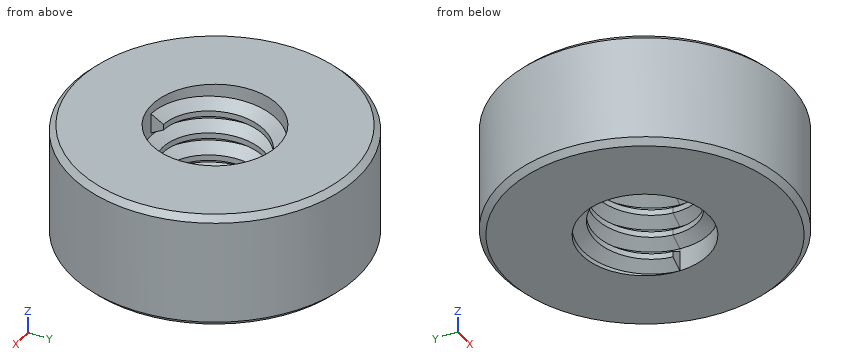
from build123d import *

# Parameters (mm, degrees)
SKETCH_1_R        = 2.5
EXTRUDE_1_DEPTH   = 2
CHAMFER_2_SIZE    = 0.1
HOLE_WIZARD_M21_D = 2.2
THREAD_1_PITCH    = 0.4
SCALE_1_SCALE     = 2


with BuildPart() as part:
    # Sketch 1 → Бобышка-Вытянуть1 (new body)
    with BuildSketch(Plane.XY):
        Circle(SKETCH_1_R)
    extrude(amount=EXTRUDE_1_DEPTH)

    # Фаска2
    chamfer_2_edges = [part.edges().sort_by_distance(p)[0] for p in [
        (-2.5, 0, 0),
        (-2.5, 0, 2),
    ]]
    chamfer(chamfer_2_edges, length=CHAMFER_2_SIZE)

    # Отверстие с зазором M21 (through all)
    with Locations(Plane(origin=(0, 0, 0), x_dir=(-1, 0, 0), z_dir=(0, 0, -1))):
        with Locations((0, 0)):
            Hole(HOLE_WIZARD_M21_D / 2)

    # Резьба1: the profile of Sketch 1 2 profile screwed along a right-hand helix of 3.75 turns, 6 arcs to a turn; built about Z, then put on its axis
    thread_1_z = Axis((0, 0, 0), (0, 0, 1))
    thread_1_corners = [(1.1003, 0, -0.000173205), (1.1003, 0, 0.350173204), (0.88349365, 0, 0.224999999), (0.88349365, 0, 0.124999999)]
    with BuildLine(mode=Mode.PRIVATE) as thread_1_profile:
        Line(thread_1_corners[0], thread_1_corners[1])
        Line(thread_1_corners[1], thread_1_corners[2])
        Line(thread_1_corners[2], thread_1_corners[3])
        Line(thread_1_corners[3], thread_1_corners[0])
    thread_1_cap = Face(thread_1_profile.wire())
    thread_1_turn_angles = [0, 30, 60, 90, 120, 150, 180, 210, 240, 270, 300, 330, 360]
    thread_1_turn_weights = [1, 0.8660254037844387, 1, 0.8660254037844387, 1, 0.8660254037844387, 1, 0.8660254037844387, 1, 0.8660254037844387, 1, 0.8660254037844387, 1]
    thread_1_turn_rails = [Edge.make_bspline([Vector(p[0], p[1], 0).rotate(thread_1_z, thread_1_turn_angles[k]) / thread_1_turn_weights[k] + Vector(0, 0, p[2] + THREAD_1_PITCH * thread_1_turn_angles[k] / 360) for k in range(13)], [0, 0, 0, 1, 1, 2, 2, 3, 3, 4, 4, 5, 5, 6, 6, 6], 2, thread_1_turn_weights) for p in thread_1_corners]
    thread_1_turn_sides = [Face.make_surface_from_curves(thread_1_turn_rails[p[0]], thread_1_turn_rails[p[1]]) for p in [(0, 1), (1, 2), (2, 3), (3, 0)]]
    thread_1_last_angles = [1080, 1110, 1140, 1170, 1200, 1230, 1260, 1290, 1320, 1335, 1350]
    thread_1_last_weights = [1, 0.8660254037844387, 1, 0.8660254037844387, 1, 0.8660254037844387, 1, 0.8660254037844387, 1, 0.9659258262890683, 1]
    thread_1_last_rails = [Edge.make_bspline([Vector(p[0], p[1], 0).rotate(thread_1_z, thread_1_last_angles[k]) / thread_1_last_weights[k] + Vector(0, 0, p[2] + THREAD_1_PITCH * thread_1_last_angles[k] / 360) for k in range(11)], [0, 0, 0, 1, 1, 2, 2, 3, 3, 4, 4, 5, 5, 5], 2, thread_1_last_weights) for p in thread_1_corners]
    thread_1_last_sides = [Face.make_surface_from_curves(thread_1_last_rails[p[0]], thread_1_last_rails[p[1]]) for p in [(0, 1), (1, 2), (2, 3), (3, 0)]]
    thread_1 = Plane(origin=(0, 0, 0), x_dir=(1, 0, 0), z_dir=(0, 0, 1)) * Solid(Shell([*[p.moved(Location((0, 0, THREAD_1_PITCH * i))) for i in range(3) for p in thread_1_turn_sides], *thread_1_last_sides, thread_1_cap, thread_1_cap.rotate(thread_1_z, 1350).moved(Location((0, 0, THREAD_1_PITCH * 1350 / 360)))]))
    add(thread_1)


with BuildPart() as part_1:
    # Масштаб1: scaled about (-0.001502253, 0.001928921, 0.997553273)
    add(part.part.scale(SCALE_1_SCALE).moved(Location((0.001502253, -0.001928921, -0.997553273))))


solid = part_1.part
The model under review builds one solid part; all positions refer to its coordinate system, in mm. Round coordinates to 2 decimals unless told otherwise and drop trailing zeros. Return JSON: item names as keys, results as strings.
(1) Add section A-A on y = -2. State how many separate pieces and enclosed holes the cut face has, plus the area to 3 significant figures.
Solved:
{"separate pieces": "1", "enclosed holes": "2", "area": "32.7 mm2"}
(2) For pin 1 (4 mm diameter, centred on x = 0, y = 0, fed in from +Z), flat-tipped, find the tip position at first contact; note if it passes through.
Solved:
{"pin 1": "z = 2.59"}
(3) For line 1 (X direction, y = 1, z = 1.1); line 2 (X direction, y = 0.75, z = -0.35); line 3 (Y direction, x = 0.25, z = -0.15), list the stretches that pass through material, from the lowest coordinate up.
Solved:
{"line 1": "-4.9 to -1.62, 1.46 to 4.9", "line 2": "-4.94 to -1.6, 1.88 to 4.94", "line 3": "-5 to -1.79, 2.12 to 4.99"}
